from build123d import *

# Parameters (mm, degrees)
SKETCH1_W           = 10.16
SKETCH1_H           = 5.08
BOSS_EXTRUDE1_DEPTH = 0.508
SKETCH2_W           = 0.6773418
SKETCH2_H           = 5.08
BOSS_EXTRUDE2_DEPTH = 0.254
CHAMFER3_SIZE       = 0.254
CHAMFER4_SIZE       = 0.254
CHAMFER5_SIZE       = 0.254


with BuildPart() as part:
    # Sketch1 → Boss-Extrude1 (new body)
    with BuildSketch(Plane.XY):
        with Locations((5.08, 2.54)):
            Rectangle(SKETCH1_W, SKETCH1_H)
    extrude(amount=BOSS_EXTRUDE1_DEPTH)

    # Sketch2 → Boss-Extrude2 (add)
    with BuildSketch(Plane.XY.offset(0.508)):
        with Locations((2.3706709, 2.54)):
            Rectangle(SKETCH2_W, SKETCH2_H)
        with Locations((5.0800127, 2.54)):
            Rectangle(SKETCH2_W, SKETCH2_H)
        with Locations((7.7893545, 2.54)):
            Rectangle(SKETCH2_W, SKETCH2_H)
    extrude(amount=BOSS_EXTRUDE2_DEPTH)

    # Chamfer3
    chamfer3_edges = [part.edges().sort_by_distance(p)[0] for p in [
        (5.08, 5.08, 0),
        (10.16, 2.54, 0),
        (5.08, 0, 0),
        (1.016, 0, 0.508),
        (3.7253418, 0, 0.508),
        (6.4346836, 0, 0.508),
        (9.1440127, 0, 0.508),
        (10.16, 2.54, 0.508),
        (9.1440127, 5.08, 0.508),
        (6.4346836, 5.08, 0.508),
        (3.7253418, 5.08, 0.508),
        (1.016, 5.08, 0.508),
    ]]
    chamfer(chamfer3_edges, length=CHAMFER3_SIZE - 0.0001)  # a hair under: the kernel refuses the full size

    # Chamfer4
    chamfer4_edges = [part.edges().sort_by_distance(p)[0] for p in [
        (0, 2.54, 0),
        (0, 2.54, 0.508),
    ]]
    chamfer(chamfer4_edges, length=CHAMFER4_SIZE - 0.0001)  # a hair under: the kernel refuses the full size

    # Chamfer5
    chamfer5_edges = [part.edges().sort_by_distance(p)[0] for p in [
        (2.3706709, 5.08, 0.762),
        (2.7093418, 2.54, 0.762),
        (2.032, 2.54, 0.762),
        (2.3706709, 0, 0.762),
        (5.4186836, 2.54, 0.762),
        (5.0800127, 5.08, 0.762),
        (4.7413418, 2.54, 0.762),
        (5.0800127, 0, 0.762),
        (8.1280254, 2.54, 0.762),
        (7.7893545, 5.08, 0.762),
        (7.4506836, 2.54, 0.762),
        (7.7893545, 0, 0.762),
    ]]
    chamfer(chamfer5_edges, length=CHAMFER5_SIZE - 0.0001)  # a hair under: the kernel refuses the full size


solid = part.part
The model under review builds one solid part; all positions refer to its coordinate system, in mm. A direction names the side the tool comes from. Give positions to 0.01 mm unless a question says otherwise; leave off trailing zeros. Order: outer loops, then holes, each group sorted by start corner. A loop starts at its lowest first (then second) coordinate and runs counter-clockwise, first axis right, second up. Notation, with made-up numbers: M 86,29 L 100,29 A21 ccw 100,35 Z; hole C -23.75,-9 d5. An arc over 180 degrees is marked long. Answer in a Markdown table with one row per item. Add a question column.
1. Mouldability with a two-part tool opening along X and no side actions: class faces 1 (the flat face through (5, 3, 0)), 2 (the flat face through (4, 3, 0.508)) as released by +X, released by -X, zero draft, split by the parting line, or undercut.
2. Add section C-C on x = 8. State the section outline as (y, z) points, plus the area to 3 significant figures.
3. To check wall thickness, follow line 1 along X through (y, z) = (4.1, 0.65); line 2 along X through (y, z) = (3.05, 0.6); line 3 along Z through (x, y) = (6.75, 1.65). State the ranges of each line that lie inside material, in increasing order.
4. For pin 1 Ø0.6 at (x, y) = (3.5, 2) entering from +Z; pin 2 Ø1.4 at (x, y) = (1.5, 2) entering from +Z, all flat-tipped, find the tip position at first contact; note any pin that passes through.
5. Machinability: for faces 3 (the flat face through (1, 3, 0.508)), 4 (the flat face through (9, 3, 0.508)), 5 (the flat face through (6, 3, 0.508)), which of the approach directions +Z, -Z, +X, -X, +Y, -Y give a long, thin tool a straight path to every point of the face, cutting with its end or side? Answer none if there is none.
The answers:
| question | item | result |
|---|---|---|
| 1 | face 1 | zero draft |
| 1 | face 2 | undercut |
| 2 | outline | M 0,0.25 L 0.25,0 L 4.83,0 L 5.08,0.25 L 5.08,0.51 L 4.95,0.64 L 0.13,0.64 L 0,0.51 Z |
| 2 | area | 3.15 mm2 |
| 3 | line 1 | 2.17 to 2.57, 4.88 to 5.28, 7.59 to 7.99 |
| 3 | line 2 | 2.12 to 2.62, 4.83 to 5.33, 7.54 to 8.04 |
| 3 | line 3 | 0 to 0.51 |
| 4 | pin 1 | z = 0.51 |
| 4 | pin 2 | z = 0.68 |
| 5 | face 3 | +Z, -X, +Y, -Y |
| 5 | face 4 | +Z, +X, +Y, -Y |
| 5 | face 5 | +Z, +Y, -Y |
